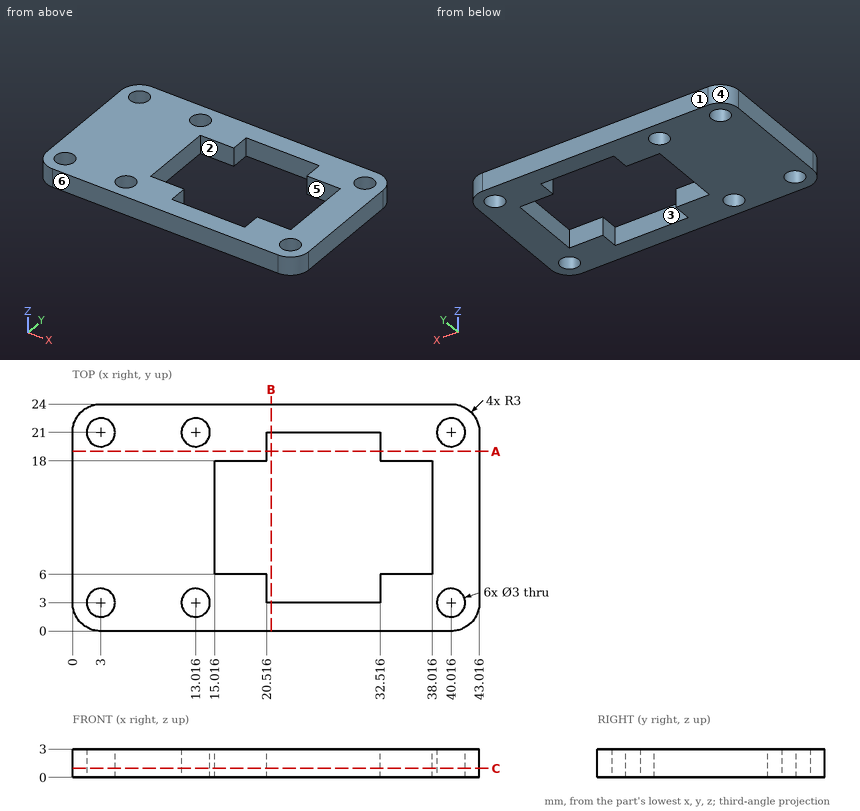
Study the drawing (mm; zero at the part's minimum x, y, z) and answer. A direction names the side the tool comes from. Round coordinates to 2 decimals unless told otherwise and drop trailing zeros. Order: outer loops, then holes, each group sorted by start corner. A loop starts at its lowest first (then second) coordinate and runs counter-clockwise, first axis right, second up. Notation, with made-up numbers: M -6,71 L 49,71 A35 cw 49,106 Z; hole C 58.25,8.25 d3. An arc over 180 degrees is marked long. One line per item, written item: value.
Q1. Straight lines are drawn through the part: line 1 (Y direction, x = 2.5, z = 1.8); line 2 (Y direction, x = 36, z = 0.55); line 3 (X direction, y = 16.25, z = 0.25). For each, find the intervals that lie inside material, in ascending order.
Derived:
line 1: 0.04 to 1.59, 4.41 to 19.59, 22.41 to 23.96
line 2: 0 to 6, 18 to 24
line 3: 0 to 15.02, 38.02 to 43.02
Q2. Flat-ended cylindrical pins translate along their axes: pin 1 (1.5 mm diameter, centred on x = 5.5, y = 13.5, fed in from -Z); pin 2 (2.5 mm diameter, centred on x = 40.02, y = 21, fed in from +Z). Find the tip coordinate at first contact, or state that the pin passes through.
Derived:
pin 1: z = 0
pin 2: through
Q3. For the marked faces 1 and 2, determine the directions among +Z, -Z, +X, -X, +Y, -Y from which every point of the face is accessible in a straight line to the end or side of a thin tool.
Derived:
face 1: +Z, -Z, +X, -X, +Y
face 2: +Z, -Z
Q4. Determine the mould class of the marked faces 3, 4, 5 and 6 for opening direction X: released by +X, released by -X, zero draft, split by the parting line, or undercut.
Derived:
face 3: undercut
face 4: released by -X
face 5: undercut
face 6: zero draft
Q5. Find section A-A on y = 19. Write down the section's boundary in (x, z).
Derived:
outline: M 0,0 L 20.52,0 L 20.52,3 L 0,3 Z; M 32.52,0 L 43.02,0 L 43.02,3 L 32.52,3 Z
Q6. Find section C-C on z = 0.95. Write down the section's boundary in (x, y), then the cut area to 3 significant figures.
Derived:
outline: M 0,3 A3 ccw 3,0 L 40.02,0 A3 ccw 43.02,3 L 43.02,21 A3 ccw 40.02,24 L 3,24 A3 ccw 0,21 Z; hole C 3,3 d3; hole C 3,21 d3; hole C 13.02,3 d3; hole C 13.02,21 d3; hole M 15.02,6 L 20.52,6 L 20.52,3 L 32.52,3 L 32.52,6 L 38.02,6 L 38.02,18 L 32.52,18 L 32.52,21 L 20.52,21 L 20.52,18 L 15.02,18 Z; hole C 40.02,3 d3; hole C 40.02,21 d3
area: 634 mm²
Q7. Find section B-B on x = 21. Write down the section's boundary in (y, z).
Derived:
outline: M 0,0 L 3,0 L 3,3 L 0,3 Z; M 21,0 L 24,0 L 24,3 L 21,3 Z
